Check sheet for the modelled part. Datum: model origin and axes. Units: mm. A direction names the side the tool comes from. Give positions to 0.01 mm unless a question says otherwise; leave off trailing zeros. Order: outer loops, then holes, each group sorted by start corner. A loop starts at its lowest first (then second) coordinate and runs counter-clockwise, first axis right, second up. Notation, with made-up numbers: M 2.25,13 L 8.25,13 A18 ccw 8.25,35 Z; hole C 59,7.5 d4. An arc over 180 degrees is marked long. One line per question, with ' | ' between items. Start each with the question number.
```python
from build123d import *

# Parameters (mm, degrees)
SKETCH1_W           = 30
SKETCH1_H           = 13
BOSS_EXTRUDE1_DEPTH = 14
SKETCH2_R           = 1.6
BOSS_EXTRUDE2_DEPTH = 1.5


with BuildPart() as part:
    # Sketch1 → Boss-Extrude1 (new body)
    with BuildSketch(Plane.XY):
        Rectangle(SKETCH1_W, SKETCH1_H)
    extrude(amount=BOSS_EXTRUDE1_DEPTH)

    # Sketch2 → Boss-Extrude2 (add)
    with BuildSketch(Plane.XY):
        with BuildLine():
            Line((15, -3.8), (15, 3.8))
            Line((15, 3.8), (18.5, 3.8))
            ThreePointArc((18.5, 3.8), (22.3, 0), (18.5, -3.8))
            Line((18.5, -3.8), (15, -3.8))
        make_face()
        with Locations((18.5, 0)):
            Circle(SKETCH2_R, mode=Mode.SUBTRACT)
    boss_extrude2 = extrude(amount=BOSS_EXTRUDE2_DEPTH)

    # Mirror1: Boss-Extrude2 across plane
    add(boss_extrude2.mirror(Plane(origin=(0, 0, 0), x_dir=(0, 0, 1), z_dir=(1, 0, 0))))


solid = part.part
```
Item 1: Set-up check for faces 1 (the face through (-17, 3.8, 1)), 2 (the face through (-17, -1, 1.5)), 3 (the face through (17, -3.8, 1)), 4 (the face through (17, 3.8, 1)): record each of +Z, -Z, +X, -X, +Y, -Y from which the full face is reachable in a straight line by a thin tool's end or side.
Item 2: Go/stop test with flat-tipped pins: P1, Ø0.8, axis at x = -17.5, z = 1, coming from the -Y side; P2, Ø4, axis at y = 2.5, z = 7.5, coming from the +X side; P3, Ø6.5, axis at y = -2.5, z = 8, coming from the -X side. Record where each tip stops, or that it passes through.
Item 3: Scan lines: probe 1 along Y at (x, z) = (-18.5, 0.6); probe 2 along X at (y, z) = (-2.75, 9.75); probe 3 along Z at (x, y) = (-16.5, -0.75). Record each from-to range of solid material in increasing order. Write a range as [from, to].
Item 4: Section check C-C, the plane y = 2.5. Record the cut outline in (x, z).
Item 5: Section check A-A, the plane y = 0. Record the cut outline in (x, z).
Item 6: Section check B-B, the plane z = 6. Record the cut outline in (x, y).
Item 7: Section check D-D, the plane y = 4.25. Record the cut outline in (x, z), then the cut area to 3 significant figures.
Item 8: Draft check along Y on faces 5 (the face through (0, 6.5, 7)), 6 (the face through (-17, -3.8, 1)), 7 (the face through (17.32, 1.08, 0.74)). Enter one of: released by +Y, released by -Y, zero draft, split by the parting line, or undercut.
Reported:
1) face 1: +Z, -Z, -X, +Y | face 2: +Z, -X, +Y, -Y | face 3: +Z, -Z, +X, -Y | face 4: +Z, -Z, +X, +Y
2) P1: stops at y = -3.8 | P2: stops at x = 15 | P3: stops at x = -15
3) probe 1: y = [-3.8, -1.6], [1.6, 3.8] | probe 2: x = [-15, 15] | probe 3: z = [0, 1.5]
4) outline: M -21.36,0 L 21.36,0 L 21.36,1.5 L 15,1.5 L 15,14 L -15,14 L -15,1.5 L -21.36,1.5 Z
5) outline: M -22.3,0 L -20.1,0 L -20.1,1.5 L -22.3,1.5 Z; M -16.9,0 L 16.9,0 L 16.9,1.5 L 15,1.5 L 15,14 L -15,14 L -15,1.5 L -16.9,1.5 Z; M 20.1,0 L 22.3,0 L 22.3,1.5 L 20.1,1.5 Z
6) outline: M -15,-6.5 L 15,-6.5 L 15,6.5 L -15,6.5 Z
7) outline: M -15,0 L 15,0 L 15,14 L -15,14 Z | area: 420 mm^2
8) face 5: released by +Y | face 6: released by -Y | face 7: undercut
